```python
from build123d import *

# Parameters (mm, degrees)
F0_R     = 8
F0_R_2   = 2.5
F1_DEPTH = 5
F3_DEPTH = 5


with BuildPart() as f1:
    # F0 (on Top) → F1 (new body)
    with BuildSketch(Plane.XY):
        Circle(F0_R)
        Circle(F0_R_2, mode=Mode.SUBTRACT)
    extrude(amount=F1_DEPTH)

    # F2 (on face) → F3 (join)
    with BuildSketch(Plane.XY.offset(5)):
        with BuildLine():
            ThreePointArc((-7.4773131729, 2.8442552126), (-7.1554071491, 3.5777295217), (-6.7617672686, 4.2753366424))
            Line((-6.7617672686, 4.2753366424), (-7.8207838354, 4.8048487661))
            Line((-7.8207838354, 4.8048487661), (-8.5363297397, 3.3737673363))
            Line((-8.5363297397, 3.3737673363), (-7.4773131729, 2.8442552126))
        make_face()
        with BuildLine():
            ThreePointArc((-7.9668552487, 0.7274733306), (-7.8541735526, 1.5205123497), (-7.6627527787, 2.2983080412))
            Line((-7.6627527787, 2.2983080412), (-8.8251883659, 2.5233473345))
            Line((-8.8251883659, 2.5233473345), (-9.1292908359, 0.952512624))
            Line((-9.1292908359, 0.952512624), (-7.9668552487, 0.7274733306))
        make_face()
        with BuildLine():
            ThreePointArc((-7.8687898433, -1.4429644491), (-7.9736434843, -0.6488525148), (-7.9985603463, 0.1517642477))
            Line((-7.9985603463, 0.1517642477), (-9.1786777557, 0.0557325966))
            Line((-9.1786777557, 0.0557325966), (-9.0489072527, -1.5389961002))
            Line((-9.0489072527, -1.5389961002), (-7.8687898433, -1.4429644491))
        make_face()
        with BuildLine():
            ThreePointArc((-7.1903499195, -3.5069741995), (-7.5050052582, -2.7703602788), (-7.7444219752, -2.0059731478))
            Line((-7.7444219752, -2.0059731478), (-8.855179859, -2.4159927833))
            Line((-8.855179859, -2.4159927833), (-8.3011078033, -3.916993835))
            Line((-8.3011078033, -3.916993835), (-7.1903499195, -3.5069741995))
        make_face()
        with BuildLine():
            ThreePointArc((-5.9815748417, -5.3123217535), (-6.482823997, -4.6875359225), (-6.9190820262, -4.0157569542))
            Line((-6.9190820262, -4.0157569542), (-7.8785547535, -4.7095229546))
            Line((-7.8785547535, -4.7095229546), (-6.941047569, -6.006087754))
            Line((-6.941047569, -6.006087754), (-5.9815748417, -5.3123217535))
        make_face()
        with BuildLine():
            ThreePointArc((-4.3316196476, -6.7258509669), (-4.9824922283, -6.2589752512), (-5.5834146978, -5.7293525212))
            Line((-5.5834146978, -5.7293525212), (-6.3208349038, -6.655695124))
            Line((-6.3208349038, -6.655695124), (-5.0690398536, -7.6521935697))
            Line((-5.0690398536, -7.6521935697), (-4.3316196476, -6.7258509669))
        make_face()
        with BuildLine():
            ThreePointArc((-2.3621792826, -7.6433048505), (-3.1146691954, -7.3687743759), (-3.8359341578, -7.0203710114))
            Line((-3.8359341578, -7.0203710114), (-4.2969122977, -8.1109664141))
            Line((-4.2969122977, -8.1109664141), (-2.8231574225, -8.7339002532))
            Line((-2.8231574225, -8.7339002532), (-2.3621792826, -7.6433048505))
        make_face()
        with BuildLine():
            ThreePointArc((-0.2185128052, -7.9970152028), (-1.0171190163, -7.9350783806), (-1.8055284813, -7.7935913996))
            Line((-1.8055284813, -7.7935913996), (-1.956064414, -8.9680010857))
            Line((-1.956064414, -8.9680010857), (-0.3690487378, -9.171424889))
            Line((-0.3690487378, -9.171424889), (-0.2185128052, -7.9970152028))
        make_face()
        with BuildLine():
            Line((2.1122796957, -8.9324971845), (1.9412704153, -7.7608935809))
            ThreePointArc((1.9412704153, -7.7608935809), (1.1554503171, -7.9161186553), (0.3580466842, -7.9919836444))
            Line((0.3580466842, -7.9919836444), (0.5290559647, -9.163587248))
            Line((0.5290559647, -9.163587248), (2.1122796957, -8.9324971845))
        make_face()
        with BuildLine():
            Line((4.4378137396, -8.0347396148), (3.9578722946, -6.9523554929))
            ThreePointArc((3.9578722946, -6.9523554929), (3.2427976615, -7.3132936032), (2.495213574, -7.6009150252))
            Line((2.495213574, -7.6009150252), (2.975155019, -8.6832991471))
            Line((2.975155019, -8.6832991471), (4.4378137396, -8.0347396148))
        make_face()
        with BuildLine():
            Line((6.4360301064, -6.5443676496), (5.6825553055, -5.6310358905))
            ThreePointArc((5.6825553055, -5.6310358905), (5.0909675506, -6.1710654995), (4.4483422056, -6.6492294006))
            Line((4.4483422056, -6.6492294006), (5.2018170066, -7.5625611597))
            Line((5.2018170066, -7.5625611597), (6.4360301064, -6.5443676496))
        make_face()
        with BuildLine():
            Line((7.9595473202, -4.5713059318), (6.988112839, -3.8943907032))
            ThreePointArc((6.988112839, -3.8943907032), (6.5636454136, -4.5736811088), (6.0733766172, -5.2071197859))
            Line((6.0733766172, -5.2071197859), (7.0448110985, -5.8840350145))
            Line((7.0448110985, -5.8840350145), (7.9595473202, -4.5713059318))
        make_face()
        with BuildLine():
            Line((8.8959960602, -2.261080618), (7.7782515209, -1.8705088285))
            ThreePointArc((7.7782515209, -1.8705088285), (7.5522116631, -2.6389579374), (7.2504599334, -3.3809511611))
            Line((7.2504599334, -3.3809511611), (8.3682044728, -3.7715229506))
            Line((8.3682044728, -3.7715229506), (8.8959960602, -2.261080618))
        make_face()
        with BuildLine():
            Line((9.1763071307, 0.215914123), (7.9946934755, 0.2913352594))
            ThreePointArc((7.9946934755, 0.2913352594), (7.9986732589, 0.1456917916), (8, 0))
            ThreePointArc((8, 0), (7.9731485852, -0.6549058236), (7.8927745906, -1.3054153602))
            Line((7.8927745906, -1.3054153602), (9.0743882458, -1.3808364965))
            Line((9.0743882458, -1.3808364965), (9.1763071307, 0.215914123))
        make_face()
        with BuildLine():
            Line((8.7798057637, 2.6769837907), (7.6214746983, 2.4316914736))
            ThreePointArc((7.6214746983, 2.4316914736), (7.8264407244, 1.6573549974), (7.9529456978, 0.8664033288))
            Line((7.9529456978, 0.8664033288), (9.1112767632, 1.1116956459))
            Line((9.1112767632, 1.1116956459), (8.7798057637, 2.6769837907))
        make_face()
        with BuildLine():
            Line((7.7357365186, 4.9406084625), (6.6861225059, 4.3926945985))
            ThreePointArc((6.6861225059, 4.3926945985), (7.0918773562, 3.70206369), (7.4265352439, 2.9743191273))
            Line((7.4265352439, 2.9743191273), (8.4761492566, 3.5222329912))
            Line((8.4761492566, 3.5222329912), (7.7357365186, 4.9406084625))
        make_face()
        with BuildLine():
            Line((6.1211063045, 6.8398310705), (5.2576252165, 6.029707877))
            ThreePointArc((5.2576252165, 6.029707877), (5.8342418272, 5.4737210654), (6.3523694296, 4.8628595116))
            Line((6.3523694296, 4.8628595116), (7.2158505176, 5.6729827051))
            Line((7.2158505176, 5.6729827051), (6.1211063045, 6.8398310705))
        make_face()
        with BuildLine():
            Line((4.0550046196, 8.2345715735), (3.4413438124, 7.2219909142))
            ThreePointArc((3.4413438124, 7.2219909142), (4.1462929515, 6.8416558493), (4.8096749823, 6.3927323239))
            Line((4.8096749823, 6.3927323239), (5.4233357894, 7.4053129832))
            Line((5.4233357894, 7.4053129832), (4.0550046196, 8.2345715735))
        make_face()
        with BuildLine():
            Line((1.6898199243, 9.0219587722), (1.3712408807, 7.8816050679))
            ThreePointArc((1.3712408807, 7.8816050679), (2.1525279564, 7.7049739388), (2.9122356685, 7.4510994767))
            Line((2.9122356685, 7.4510994767), (3.2308147121, 8.591453181))
            Line((3.2308147121, 8.591453181), (1.6898199243, 9.0219587722))
        make_face()
        with BuildLine():
            Line((0.8, 9.1439177306), (-0.0797977611, 9.1439177306))
            Line((-0.0797977611, 9.1439177306), (-0.9594615248, 9.1285631425))
            Line((-0.9594615248, 9.1285631425), (-0.9387975573, 7.9447252405))
            ThreePointArc((-0.9387975573, 7.9447252405), (-0.069812284, 7.9996953845), (0.8, 7.9598994969))
            Line((0.8, 7.9598994969), (0.8, 9.1439177306))
        make_face()
        with BuildLine():
            ThreePointArc((-4.9205110082, 6.3078182772), (-4.2650648096, 6.7682510422), (-3.5668607998, 7.1608312391))
            Line((-3.5668607998, 7.1608312391), (-4.1981001127, 8.1625478197))
            Line((-4.1981001127, 8.1625478197), (-5.5517503211, 7.3095348578))
            Line((-5.5517503211, 7.3095348578), (-4.9205110082, 6.3078182772))
        make_face()
        with BuildLine():
            ThreePointArc((-6.4362705336, 4.7512547414), (-5.9288828486, 5.3710658316), (-5.3620573673, 5.9370313111))
            Line((-5.3620573673, 5.9370313111), (-6.2395455422, 6.7319612961))
            Line((-6.2395455422, 6.7319612961), (-7.3137587085, 5.5461847263))
            Line((-7.3137587085, 5.5461847263), (-6.4362705336, 4.7512547414))
        make_face()
        with BuildLine():
            ThreePointArc((-3.0418317373, 7.3991391176), (-2.2866704527, 7.6662336412), (-1.5085850091, 7.8564732081))
            Line((-1.5085850091, 7.8564732081), (-1.8470174479, 8.9910932601))
            Line((-1.8470174479, 8.9910932601), (-3.3802641762, 8.5337591696))
            Line((-3.3802641762, 8.5337591696), (-3.0418317373, 7.3991391176))
        make_face()
    extrude(amount=-F3_DEPTH)


solid = f1.part
```
The listing builds one solid part. Answer for the finished solid, in the listing's coordinates (mm). A direction names the side the tool comes from. Round coordinates to 2 decimals unless told otherwise and drop trailing zeros. Loops run counter-clockwise (first coordinate to the right, second up) from the corner with the lowest first, then second, coordinate; pieces in that order, holes last.
Q1. Which of the six approach directions +Z, -Z, +X, -X, +Y, -Y give full straight-line access (tool end or side, diameter ignored) to faces 1 (the face through (7.802, -3.574, 2.535)), 2 (the face through (-2.596, -8.196, 2.535)), 3 (the face through (-4.87, 7.74, 2.54))?
Q2. For a pull along Y with two mould halves and no side action, classify faces 4 (the face through (4.82, -7.1, 2.54)), 5 (the face through (6.676, 6.248, 2.535)), 6 (the face through (-7.284, 4.536, 2.535)) as released by +Y, released by -Y, zero draft, split by the parting line, or undercut.
Q3. Find the intervals of material crossed by line 1 (Y direction, x = 0, z = 2.25); line 2 (X direction, y = 6.5, z = 3.3); line 3 (Y direction, x = 0.75, z = 2.3), in increasing order.
Q4. Section B-B, the plane y = -6.25 is taken. Determine the outline of the cut face in (x, z), then the cut area to 3 significant figures.
Q5. Given pin 1 Ø3 at (y, z) = (3, 2) entering from -X; pin 2 Ø1 at (x, z) = (3.5, 3) entering from -Y; pin 3 Ø1.3 at (y, z) = (8.5, 3) entering from +X, each flat-ended and moving along its own axis, determine where each tip first touches the part or whether it passes through.
Q6. Section A-A, the plane y = 2 is taken. Determine the outline of the cut face in (x, z), then the cut area to 3 significant figures.
Completed:
1. face 1: +Z, -Z
1. face 2: +Z, -Z, -Y
1. face 3: +Z, -Z, -X, +Y
2. face 4: released by -Y
2. face 5: released by +Y
2. face 6: undercut
3. line 1: y = -8 to -2.5, 2.5 to 9.14
3. line 2: x = -6.45 to -5.98, -5.04 to 4.87, 5.76 to 6.44
3. line 3: y = -9.13 to -2.38, 2.38 to 9.14
4. outline: (-6, 0) - (6.19, 0) - (6.19, 5) - (-6, 5) - close
4. area: 61.0 mm2
5. pin 1: stops at x = -9.02
5. pin 2: stops at y = -8.67
5. pin 3: stops at x = 4.69
6. outline: (-8.93, 0) - (-1.5, 0) - (-1.5, 5) - (-8.93, 5) - close; (1.5, 0) - (8.92, 0) - (8.92, 5) - (1.5, 5) - close
6. area: 74.2 mm2
